```python
from build123d import *

# Parameters (mm, degrees)
ESQUISSE1_R        = 1.5
BOSS_EXTRU_1_DEPTH = 5


with BuildPart() as part:
    # Esquisse1 → Boss.-Extru.1 (new body)
    with BuildSketch(Plane.XY):
        with BuildLine():
            ThreePointArc((-25.5, 44.167295593), (-44.167295593, 25.5), (-51, 0))
            ThreePointArc((-51, 0), (-45, -6), (-39, 0))
            ThreePointArc((-39, 0), (-33.774990748, 19.5), (-19.5, 33.774990748))
            ThreePointArc((-19.5, 33.774990748), (-17.303847577, 41.97114317), (-25.5, 44.167295593))
        make_face()
        with Locations((-22.5, 38.97114317)):
            Circle(ESQUISSE1_R, mode=Mode.SUBTRACT)
        with Locations((-45, 0)):
            Circle(ESQUISSE1_R, mode=Mode.SUBTRACT)
        Polygon((-30.940054257, 29.410254038), (-34.690054257, 22.915063509), (-39.020181276, 25.415063509), (-35.270181276, 31.910254038), align=None, mode=Mode.SUBTRACT)
        Polygon((-45.270181276, 14.589745962), (-40.940054257, 12.089745962), (-37.190054257, 18.584936491), (-41.520181276, 21.084936491), align=None, mode=Mode.SUBTRACT)
    extrude(amount=BOSS_EXTRU_1_DEPTH)


solid = part.part
```
CAD build for the part. Positions are in the model's coordinates, mm. A direction names the side the tool comes from. Round coordinates to 2 decimals unless told otherwise and drop trailing zeros. Order: outer loops, then holes, each group sorted by start corner. A loop starts at its lowest first (then second) coordinate and runs counter-clockwise, first axis right, second up. Notation, with made-up numbers: (-15.75, 38.25) - (-2.75, 38.25) arc R34 ccw to (-2.75, 75.25) - close; hole circle Ø9 at (55.5, 42.5). An arc over 180 degrees is marked (long way). Use CSV: the item, a comma, the result in double quotes. Start each with the question number.
1) Saw through at B-B (y = 27.5). List the corners of the cut face in (x, z).
2) Tool access for faces 1 (the flat face through (-32.79, 26.21, 2.46)), 2 (the cylindrical face through (-43.98, 25.82, 2.46)): list every direction of +Z, -Z, +X, -X, +Y, -Y with a clear straight run to the whole face (end or side of a thin tool).
3) Pin check, flat tips, straight feed: pin 1 Ø1.5 at (y, z) = (8.5, 3) entering from -X; pin 2 Ø2 at (x, z) = (-37.5, 2.5) entering from +Y. Stop position of each tip, or through.
4) Saw through at A-A (x = -32). List the corners of the cut face in (y, z), and give its area (3 significant figures).
5) Two-plate mould, pull along X, no slides. Class faces 3 (the flat face through (-39.091, 15.292, 2.465)), 4 (the flat face through (-36, 21, 0)), 5 (the flat face through (-36.825, 24.148, 2.465)), 6 (the cylindrical face through (-17.24, 41.86, 2.46)): pulls with the +X half, pulls with the -X half, needs draft (parallel to the pull), parting line crosses it, or undercut.
6) Wall check: L1, parallel to Y at x = -45, z = 3; L2, parallel to X at y = 13, z = 4.3; L3, parallel to X at y = 1, z = 2.25. Give the ranges that are in metal, low to high. Write a range as [from, to].
7) Saw through at C-C (z = 0.9). List the corners of the cut face in (x, y) (3 decimals), and give its area (3 significant figures).
Values follow:
1,outline,"(-42.95, 0) - (-37.82, 0) - (-37.82, 5) - (-42.95, 5) - close; (-32.04, 0) - (-27.65, 0) - (-27.65, 5) - (-32.04, 5) - close"
2,face 1,"+Z, -Z"
2,face 2,"+Z, -Z, -X, +Y"
3,pin 1,"stops at x = -50.41"
3,pin 2,"stops at y = 35.62"
4,outline,"(22.29, 0) - (27.57, 0) - (27.57, 5) - (22.29, 5) - close; (30.02, 0) - (39.71, 0) - (39.71, 5) - (30.02, 5) - close"
4,area,"74.9 mm2"
5,face 3,"undercut"
5,face 4,"needs draft"
5,face 5,"undercut"
5,face 6,"parting line crosses it"
6,L1,"y = [-6, -1.5], [1.5, 14.43], [15.06, 24]"
6,L2,"x = [-49.32, -42.52], [-40.41, -36.77]"
6,L3,"x = [-50.99, -46.12], [-43.88, -38.99]"
7,outline,"(-51, 0) arc R6 ccw to (-39, 0) arc R39 cw to (-19.5, 33.775) arc R6 ccw to (-25.5, 44.167) arc R51 ccw to start; hole circle Ø3 at (-45, 0); hole (-45.27, 14.59) - (-40.94, 12.09) - (-37.19, 18.585) - (-41.52, 21.085) - close; hole (-39.02, 25.415) - (-34.69, 22.915) - (-30.94, 29.41) - (-35.27, 31.91) - close; hole circle Ø3 at (-22.5, 38.971)"
7,area,"589 mm2"
